For this review, take the finished solid that the model builds, in its own axes (mm). Round coordinates to 2 decimals unless told otherwise and drop trailing zeros. Write each loop counter-clockwise with the first axis right and the second up, starting at its lowest first coordinate (ties: lowest second). Pieces come first, ordered by that corner, then holes. Notation, with made-up numbers: (-25.75, -35) - (3.25, -35) arc R24 ccw to (3.25, 3) - close; hole circle Ø2 at (-34, 67). An arc over 180 degrees is marked (long way). Answer in a Markdown table with one row per item. Add a question column.
Autodesk Inventor part; units mm, degrees
ref_plane "YZ Plane" through (0, 0, 0) normal (1, 0, 0) x (0, 1, 0)
ref_plane "XZ Plane" through (0, 0, 0) normal (0, 1, 0) x (-1, 0, 0)
ref_plane "XY Plane" through (0, 0, 0) normal (0, 0, 1) x (1, 0, 0)
sketch "Sketch1" plane through (0, 0, 0) normal (0, 0, 1) x (1, 0, 0)
  circle A0 centre (0, 0) radius 5.9
  circle A1 centre (0, 0) radius 10
  dimension "d0" = 11.8
  dimension "d1" = 20
extrude "Extrusion1" add sketch "Sketch1" along normal mid plane 60
thread "Thread1"
thread "Thread2"
chamfer "Chamfer1" distance 1 angle 45 2 edges at (-5.9, 0, 30) (-5.9, 0, -30)
fillet "Fillet1" radius 2 2 edges at (-10, 0, -30) (-10, 0, 30)
properties part number "Plenum"
Q1. To check wall thickness, follow probe 1 along Y at (x, z) = (0, 8.5); probe 2 along X at (y, z) = (2.5, 25); probe 3 along Y at (x, z) = (4.25, 5.5). State the ranges of each line that lie inside material, in increasing order.
Q2. Add section C-C on z = -22. State the section outline as (x, y) points, then the cut area to 3 significant figures.
Q3. Insertion check: pin 1 Ø12 at (y, z) = (8, 0.5) entering from -X; pin 2 Ø1.5 at (y, z) = (3.5, 5.5) entering from +X; pin 3 Ø12 at (x, z) = (-7.5, -1) entering from +Y. Each pin has a flat end and moves straight along its axis. Give the tip position at first contact, or say it passes through.
Q4. Add section A-A on y = 0. State the section outline as (x, z) points.
Q5. Draft analysis for pull direction X (two halves, no side actions). For faces 1 (the face through (-6, -4, -30)), 2 (the face through (-2.17, -9.76, 0.39)), 3 (the face through (-5.894, 0.259, 0.406)), state which applies: released by +X, released by -X, zero draft, split by the parting line, or undercut.
Answer sheet:
| question | item | result |
|---|---|---|
| 1 | probe 1 | y = -10 to -5.9, 5.9 to 10 |
| 1 | probe 2 | x = -9.68 to -5.34, 5.34 to 9.68 |
| 1 | probe 3 | y = -9.05 to -4.09, 4.09 to 9.05 |
| 2 | outline | circle Ø20 at (0, 0); hole circle Ø11.8 at (0, 0) |
| 2 | area | 205 mm² |
| 3 | pin 1 | stops at x = -9.8 |
| 3 | pin 2 | stops at x = 9.61 |
| 3 | pin 3 | stops at y = 9.89 |
| 4 | outline | (-10, -28) arc R2 ccw to (-8, -30) - (-6.9, -30) - (-5.9, -29) - (-5.9, 29) - (-6.9, 30) - (-8, 30) arc R2 ccw to (-10, 28) - close; (5.9, -29) - (6.9, -30) - (8, -30) arc R2 ccw to (10, -28) - (10, 28) arc R2 ccw to (8, 30) - (6.9, 30) - (5.9, 29) - close |
| 5 | face 1 | zero draft |
| 5 | face 2 | split by the parting line |
| 5 | face 3 | undercut |
